from build123d import *

# Parameters (mm, degrees)
BOSS_EXTRUDE1_DEPTH     = 30
CUT_EXTRUDE1_DEPTH      = 197.169807399
SKETCH4_W               = 32
SKETCH4_H               = 68.5
CUT_EXTRUDE2_DEPTH      = 197.169807399
CHAMFER1_SIZE           = 7.802060087
CHAMFER1_SIZE_2         = 10
CUT_EXTRUDE3_DEPTH      = 163.649773439
CUT_EXTRUDE4_DEPTH      = 181.083572192
CUT_EXTRUDE4_DEPTH_BACK = 181.083572192
SKETCH6_R               = 2
FILL_PATTERN1_DEPTH     = 8
FILLET5_R               = 20
FILLET2_R               = 5
FILLET4_R               = 2
FILLET6_R               = 2


# Read off the part's stored shape, not the designer's step: Fill Pattern1
with BuildPart() as part:
    # Sketch2 → Boss-Extrude1 (new, symmetric)
    with BuildSketch(Plane(origin=(0, 0, 0), x_dir=(0, 0, -1), z_dir=(1, 0, 0))):
        Polygon((35.163005932, 120), (-52.189850292, -120), (-52.189850292, -168.5), (-39.189850292, -168.5), (-39.189850292, -162.5), (-40.589850292, -162.5), (-40.589850292, -164.5), (-47.189850292, -164.5), (-47.189850292, -124), (-40.589850292, -124), (-40.589850292, -139), (-36.589850292, -139), (-36.589850292, -120), (-43.676428112, -120), (43.676428112, 120), align=None)
    extrude(amount=BOSS_EXTRUDE1_DEPTH, both=True)

    # Sketch3 → Cut-Extrude1 (cut, through all)
    with BuildSketch(Plane.XY.offset(52.189850292)):
        Polygon((-30, 120), (-30, -120), (-10, 120), align=None)
        Polygon((10, 120), (30, 120), (30, -120), align=None)
    extrude(amount=-CUT_EXTRUDE1_DEPTH, mode=Mode.SUBTRACT)

    # Sketch4 → Cut-Extrude2 (cut, through all)
    with BuildSketch(Plane.XY.offset(52.189850292)):
        with Locations((0, -134.25)):
            Rectangle(SKETCH4_W, SKETCH4_H)
    extrude(amount=-CUT_EXTRUDE2_DEPTH, mode=Mode.SUBTRACT)

    # Chamfer1
    # the kernel refuses this chamfer: 10, 7.802060087 mm, written as the material it adds along each edge
    with BuildSketch(Plane(origin=(-16, -120, 43.676428112), x_dir=(0, 0.9542611885293295, -0.29897421973573485), z_dir=(-1, 0, 0))) as chamfer1_piece_1_section:
        Polygon((CHAMFER1_SIZE * 0.998967402661, CHAMFER1_SIZE * 0.0454326803806), (CHAMFER1_SIZE_2 * 0.298974219736, CHAMFER1_SIZE_2 * 0.954261188529), (0, 0), align=None)
    chamfer1_piece_1 = extrude(amount=14, mode=Mode.PRIVATE)
    chamfer1_piece_1 = split(chamfer1_piece_1, bisect_by=Plane(origin=(-29.733836006, -116.806032072, 40.079574986), z_dir=(0.9965457582448797, -0.08304547985373997, 0)), keep=Keep.TOP, mode=Mode.PRIVATE)
    chamfer1_piece_1 = split(chamfer1_piece_1, bisect_by=Plane(origin=(-22.890520375, -117.376308375, 36.589850292), z_dir=(0, 0, 1)), keep=Keep.TOP, mode=Mode.PRIVATE)
    add(chamfer1_piece_1)
    with BuildSketch(Plane(origin=(30, -120, 43.676428112), x_dir=(0, 0.9542611885293295, -0.29897421973573485), z_dir=(-1, 0, 0))) as chamfer1_piece_2_section:
        Polygon((CHAMFER1_SIZE * 0.998967402661, CHAMFER1_SIZE * 0.0454326803806), (CHAMFER1_SIZE_2 * 0.298974219736, CHAMFER1_SIZE_2 * 0.954261188529), (0, 0), align=None)
    chamfer1_piece_2 = extrude(amount=14, mode=Mode.PRIVATE)
    chamfer1_piece_2 = split(chamfer1_piece_2, bisect_by=Plane(origin=(29.733836006, -116.806032072, 40.079574986), z_dir=(-0.9965457582448797, -0.08304547985373997, 0)), keep=Keep.TOP, mode=Mode.PRIVATE)
    chamfer1_piece_2 = split(chamfer1_piece_2, bisect_by=Plane(origin=(22.890520375, -117.376308375, 36.589850292), z_dir=(0, 0, 1)), keep=Keep.TOP, mode=Mode.PRIVATE)
    add(chamfer1_piece_2)

    # Sketch5 → Cut-Extrude3 (cut, through all)
    with BuildSketch(Plane(origin=(0, -20.133671251, 15.841479222), x_dir=(1, 0, 0), z_dir=(0, 0.3420201433256661, 0.9396926207859094))):
        Polygon((6.25, 149.12713812), (6.25, 136.62713812), (-6.25, 136.62713812), (-6.25, 149.12713812), (-6.25, 152.038899995), (6.25, 152.038899995), align=None)
    extrude(amount=-CUT_EXTRUDE3_DEPTH, mode=Mode.SUBTRACT)

    # Sketch6 → Cut-Extrude4 (cut, two sides: drawn at the far end of the back side and taken through both)
    with BuildSketch(Plane.ZY.offset(-6.25).offset(-CUT_EXTRUDE4_DEPTH_BACK)):
        with Locations(Location((-37.211675699, 113.933456323, 0), (0, 0, 270))):
            Circle(SKETCH6_R)
    extrude(amount=CUT_EXTRUDE4_DEPTH + CUT_EXTRUDE4_DEPTH_BACK, mode=Mode.SUBTRACT)

    # Fill Pattern1 outline → Fill Pattern1 (cut)
    with BuildSketch(Plane(origin=(0, 0, 0), x_dir=(1, 0, 0), z_dir=(0, 0.34202014332566616, 0.9396926207859093))):
        Polygon((8.5, -84.523921196), (15.42820323, -80.523921196), (15.42820323, -72.523921196), (8.5, -68.523921196), (1.57179677, -72.523921196), (1.57179677, -80.523921196), align=None)
        Polygon((15.42820323, -51.079057467), (15.42820323, -43.079057467), (8.5, -39.079057467), (1.57179677, -43.079057467), (1.57179677, -51.079057467), (8.5, -55.079057467), align=None)
        Polygon((15.42820323, -21.634193738), (15.42820323, -13.634193738), (8.5, -9.634193738), (1.57179677, -13.634193738), (1.57179677, -21.634193738), (8.5, -25.634193738), align=None)
        Polygon((-8.5, -25.634193738), (-1.57179677, -21.634193738), (-1.57179677, -13.634193738), (-8.5, -9.634193738), (-15.42820323, -13.634193738), (-15.42820323, -21.634193738), align=None)
        Polygon((-1.57179677, -51.079057467), (-1.57179677, -43.079057467), (-8.5, -39.079057467), (-15.42820323, -43.079057467), (-15.42820323, -51.079057467), (-8.5, -55.079057467), align=None)
        Polygon((-1.57179677, -80.523921196), (-1.57179677, -72.523921196), (-8.5, -68.523921196), (-15.42820323, -72.523921196), (-15.42820323, -80.523921196), (-8.5, -84.523921196), align=None)
        Polygon((0, -40.356625603), (6.92820323, -36.356625603), (6.92820323, -28.356625603), (0, -24.356625603), (-6.92820323, -28.356625603), (-6.92820323, -36.356625603), align=None)
        Polygon((6.92820323, -6.911761874), (6.92820323, 1.088238126), (0, 5.088238126), (-6.92820323, 1.088238126), (-6.92820323, -6.911761874), (0, -10.911761874), align=None)
        Polygon((6.92820323, 22.533101855), (6.92820323, 30.533101855), (0, 34.533101855), (-6.92820323, 30.533101855), (-6.92820323, 22.533101855), (0, 18.533101855), align=None)
        Polygon((6.92820323, 81.422829312), (6.92820323, 89.422829312), (0, 93.422829312), (-6.92820323, 89.422829312), (-6.92820323, 81.422829312), (0, 77.422829312), align=None)
        Polygon((6.92820323, 51.977965583), (6.92820323, 59.977965583), (0, 63.977965583), (-6.92820323, 59.977965583), (-6.92820323, 51.977965583), (0, 47.977965583), align=None)
        Polygon((6.92820323, -65.801489331), (6.92820323, -57.801489331), (0, -53.801489331), (-6.92820323, -57.801489331), (-6.92820323, -65.801489331), (0, -69.801489331), align=None)
        Polygon((6.92820323, -95.24635306), (6.92820323, -87.24635306), (0, -83.24635306), (-6.92820323, -87.24635306), (-6.92820323, -95.24635306), (0, -99.24635306), align=None)
    extrude(amount=FILL_PATTERN1_DEPTH, mode=Mode.SUBTRACT)

    # Fillet5
    fillet5_edges = [part.edges().sort_by_distance(p)[0] for p in [
        (23, -120, 52.189850292),
        (-23, -120, 52.189850292),
    ]]
    fillet(fillet5_edges, radius=FILLET5_R)

    # Fillet2
    fillet2_edges = [part.edges().sort_by_distance(p)[0] for p in [
        (-16, -100, 40.653734517),
        (16, -100, 40.653734517),
    ]]
    fillet(fillet2_edges, radius=FILLET2_R)

    # Fillet4
    fillet4_edges = [part.edges().sort_by_distance(p)[0] for p in [
        (-8.125, 120, -43.676428112),
        (-8.125, 120, -35.163005932),
        (8.125, 120, -43.676428112),
        (8.125, 120, -35.163005932),
    ]]
    fillet(fillet4_edges, radius=FILLET4_R)

    # Fillet6
    fillet6_edges = [part.edges().sort_by_distance(p)[0] for p in [
        (23, -168.5, 39.189850292),
        (23, -168.5, 52.189850292),
        (-23, -168.5, 39.189850292),
        (-23, -168.5, 52.189850292),
    ]]
    fillet(fillet6_edges, radius=FILLET6_R)


solid = part.part
Here's how the part is built. I have some questions about the finished solid (model axes, mm). A direction names the side the tool comes from. Round coordinates to 2 decimals unless told otherwise and drop trailing zeros. Loops run counter-clockwise (first coordinate to the right, second up) from the corner with the lowest first, then second, coordinate; pieces in that order, holes last. Notation, with made-up numbers: (73, -30.5) -> (91, -30.5) arc R13 cw to (91, -9.5) -> close; hole circle Ø10 at (4, 62). An arc over 180 degrees is marked (long way). Write each question's results on one line, items separated by ' | '.
(1) If we section it at B-B, the plane x = -24.5: List the corners of the cut face in (y, z) for me.
Worked answers:
outline: (-168.5, 41.19) arc R2 ccw to (-166.5, 39.19) -> (-162.5, 39.19) -> (-162.5, 40.59) -> (-164.5, 40.59) -> (-164.5, 47.19) -> (-124, 47.19) -> (-124, 40.59) -> (-139, 40.59) -> (-139, 36.59) -> (-117.09, 36.59) -> (-112.67, 41.01) -> (-54, 19.65) -> (-54, 28.17) -> (-116.69, 50.98) arc R20 ccw to (-123.53, 52.19) -> (-166.5, 52.19) arc R2 ccw to (-168.5, 50.19) -> close
(2) For P1, Ø3, axis at x = 11.5, y = -90.5, coming from the +Z side; P2, Ø15.5, axis at x = -23.5, y = -132.5, coming from the -Z side; P3, Ø2, axis at x = -20, z = 38, coming from the -Y side; P4, Ø2, axis at x = -3.5, y = 0.5, coming from the -Z side, each with a flat end and sliding along its axis, tell me the tip position at first contact or that it passes through.
Worked answers:
P1: z = 42 | P2: z = 36.59 | P3: y = -139 | P4: through
(3) If we section it at A-A, the plane y = -131.5: List the corners of the cut face in (x, z) for me.
Worked answers:
outline: (-30, 36.59) -> (-16, 36.59) -> (-16, 40.59) -> (-30, 40.59) -> close; (-30, 47.19) -> (-16, 47.19) -> (-16, 52.19) -> (-30, 52.19) -> close; (16, 36.59) -> (30, 36.59) -> (30, 40.59) -> (16, 40.59) -> close; (16, 47.19) -> (30, 47.19) -> (30, 52.19) -> (16, 52.19) -> close
(4) If we section it at C-C, the plane x = 21: List the corners of the cut face in (y, z) for me.
Worked answers:
outline: (-168.5, 41.19) arc R2 ccw to (-166.5, 39.19) -> (-162.5, 39.19) -> (-162.5, 40.59) -> (-164.5, 40.59) -> (-164.5, 47.19) -> (-124, 47.19) -> (-124, 40.59) -> (-139, 40.59) -> (-139, 36.59) -> (-117.09, 36.59) -> (-112.67, 41.01) -> (-12, 4.37) -> (-12, 12.88) -> (-116.69, 50.98) arc R20 ccw to (-123.53, 52.19) -> (-166.5, 52.19) arc R2 ccw to (-168.5, 50.19) -> close
(5) We'd pull the mould along X, two halves only. Please class faces 5 (the face through (-23, -168.5, 46)), 6 (the face through (-6.928, -1, 5)): released by +X, released by -X, zero draft, split by the parting line, or undercut.
Worked answers:
face 5: zero draft | face 6: undercut
(6) If I drill on L1, parallel to Z at x = -21, y = -132.5; L2, parallel to Z at x = 17.5, y = -143.5; L3, parallel to Z at x = -14, y = 4, over which ranges is the centre line in solid material (lowest first)?
Worked answers:
L1: 36.59 to 40.59, 47.19 to 52.19 | L2: 47.19 to 52.19 | L3: -1.46 to 7.06
(7) For faces 1 (the face through (23.1, -120.01, 51.88)), 2 (the face through (-12.013, -76.172, 31.921)), 3 (the face through (-6.928, 82, -26)), 4 (the face through (-11.916, -64.896, 27.817)), which set-ups out of +Z, -Z, +X, -X, +Y, -Y let a thin tool reach every point of the face, with its end or its side?
Worked answers:
face 1: +Z, +X, -X, +Y | face 2: -Z | face 3: none | face 4: +Z
(8) If we section it at D-D, the plane y = 94: List the corners of the cut face in (x, z) for me, then the cut area to 3 significant figures.
Worked answers:
outline: (-12.17, -34.21) -> (12.17, -34.21) -> (12.17, -25.7) -> (-12.17, -25.7) -> close | area: 207 mm2
